Check sheet for the modelled part. Datum: model origin and axes. Units: mm. Coordinates: 2 decimals unless noted, no trailing zeros. Order: outer loops, then holes, each group sorted by start corner. A loop starts at its lowest first (then second) coordinate and runs counter-clockwise, first axis right, second up.
from build123d import *

# Parameters (mm, degrees)
SKETCH1_R           = 5.7
BOSS_EXTRUDE1_DEPTH = 8.4


with BuildPart() as part:
    # Sketch1 → Boss-Extrude1 (new body)
    with BuildSketch(Plane(origin=(0, 0, 0), x_dir=(1, 0, 0), z_dir=(0, 1, 0))):
        Polygon((8.659137602, 0), (6.122934918, 6.122934918), (0, 8.659137602), (-6.122934918, 6.122934918), (-8.659137602, 0), (-6.122934918, -6.122934918), (0, -8.659137602), (6.122934918, -6.122934918), align=None)
        Circle(SKETCH1_R, mode=Mode.SUBTRACT)
    extrude(amount=BOSS_EXTRUDE1_DEPTH)


solid = part.part
(1) Go/stop test with a flat-tipped pin: P1, Ø3, axis at y = 1.5, z = -2, coming from the -X side. Record where the tip stops, or that it passes through.
Filled in:
P1: stops at x = -8.45
(2) Cross-section at C-C (x = -3.75). Enter the section's corners in (y, z), and give its area (3 significant figures).
Filled in:
outline: (0, -7.11) - (8.4, -7.11) - (8.4, -4.29) - (0, -4.29) - close; (0, 4.29) - (8.4, 4.29) - (8.4, 7.11) - (0, 7.11) - close
area: 47.3 mm2
(3) Thickness scan on probe 1 along X at (y, z) = (1.25, -1.25); probe 2 along X at (y, z) = (6.5, -3); probe 3 along Z at (x, y) = (-4.5, 3.25). Record the ranges inside material, lowest first.
Filled in:
probe 1: x = -8.14 to -5.56, 5.56 to 8.14
probe 2: x = -7.42 to -4.85, 4.85 to 7.42
probe 3: z = -6.8 to -3.5, 3.5 to 6.8
(4) Cross-section at D-D (z = 7.5). Enter the section's corners in (x, y), and give its area (3 significant figures).
Filled in:
outline: (-2.8, 0) - (2.8, 0) - (2.8, 8.4) - (-2.8, 8.4) - close
area: 47.0 mm2
(5) Cross-section at B-B (z = -3.5). Enter the section's corners in (x, y).
Filled in:
outline: (-7.21, 0) - (-4.5, 0) - (-4.5, 8.4) - (-7.21, 8.4) - close; (4.5, 0) - (7.21, 0) - (7.21, 8.4) - (4.5, 8.4) - close
(6) Cross-section at A-A (y = 2.25). Enter the section's corners in (x, z), and give its area (3 significant figures).
Filled in:
outline: (-8.66, 0) - (-6.12, -6.12) - (0, -8.66) - (6.12, -6.12) - (8.66, 0) - (6.12, 6.12) - (0, 8.66) - (-6.12, 6.12) - close; hole circle Ø11.4 at (0, 0)
area: 110 mm2
(7) Release check for a two-part mould opening along Z. For faces 1 (the flat face through (0, 8.4, -6)), 2 (the flat face through (7.41, 4.14, -3.02)), 3 (the cylindrical face through (-4.5, 4.1, 3.5)), 4 (the flat face through (-3.104, 4.141, 7.373)) record: +Z half, -Z half, draft (parallel to the pull), parting line (faces both ways), or undercut.
Filled in:
face 1: draft
face 2: -Z half
face 3: undercut
face 4: +Z half
